Build history of the part. All positions in model axes, mm. Give positions to 0.01 mm unless a question says otherwise; leave off trailing zeros. Write each loop counter-clockwise with the first axis right and the second up, starting at its lowest first coordinate (ties: lowest second). Pieces come first, ordered by that corner, then holes. Notation, with made-up numbers: M 67.5,48 L 113.5,48 A27 ccw 113.5,80 Z; hole C 50.25,65 d8. An arc over 180 degrees is marked long. One line per item, written item: value. Start each with the question number.
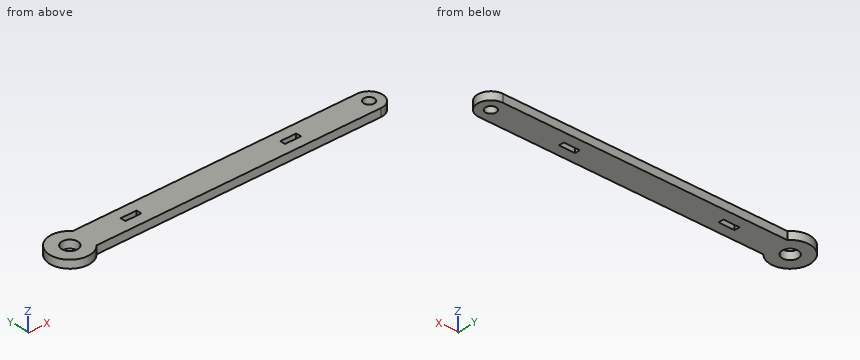
from build123d import *

# Parameters (mm, degrees)
SKETCH_1_R      = 2
SKETCH_1_R_2    = 3
SKETCH_1_W      = 6
SKETCH_1_H      = 2
EXTRUDE_1_DEPTH = 1.5


with BuildPart() as part:
    # 草图1 → 凸台-拉伸1 (new, symmetric)
    with BuildSketch(Plane.XY):
        with BuildLine():
            Line((5.590169944, 5), (112.5, 5))
            ThreePointArc((112.5, 5), (117.5, 0), (112.5, -5))
            Line((112.5, -5), (5.590169944, -5))
            ThreePointArc((5.590169944, -5), (-7.5, 0), (5.590169944, 5))
        make_face()
        with Locations((112.5, 0)):
            Circle(SKETCH_1_R, mode=Mode.SUBTRACT)
        Circle(SKETCH_1_R_2, mode=Mode.SUBTRACT)
        with Locations((23, 0)):
            Rectangle(SKETCH_1_W, SKETCH_1_H, mode=Mode.SUBTRACT)
        with Locations((83, 0)):
            Rectangle(SKETCH_1_W, SKETCH_1_H, mode=Mode.SUBTRACT)
    extrude(amount=EXTRUDE_1_DEPTH, both=True)


solid = part.part
1) Drop flat-ended pins along their axis: P1, Ø0.9, axis at x = 23, z = 0, coming from the -Y side; P2, Ø0.6, axis at y = -0.5, z = -0.5, coming from the +X side; P3, Ø0.9, axis at x = 84, z = 0, coming from the +Y side. Give the stop position or say it passes through.
2) Probe line 1 along Y through (x, z) = (112.5, 0.1); line 2 along Y through (x, z) = (0, 0.2); line 3 along X through (y, z) = (-1.25, 1.05). List the from-to ranges inside material, lowest first. Write a range as from..to.
3) Band-saw the part on B-B (z = -0.35). List the corners of the cut face in (x, y).
4) Band-saw the part on C-C (x = 14.5). List the corners of the cut face in (y, z).
5) Band-saw the part on A-A (x = 0). List the corners of the cut face in (y, z), then the cut area to 3 significant figures.
Model answer:
1. P1: stops at y = -5
1. P2: stops at x = 117.5
1. P3: stops at y = 5
2. line 1: y = -5..-2, 2..5
2. line 2: y = -7.5..-3, 3..7.5
2. line 3: x = -7.4..-2.73, 2.73..110.94, 114.06..117.34
3. outline: M 5.59,-5 L 112.5,-5 A5 ccw 112.5,5 L 5.59,5 A7.5 ccw long Z; hole C 0,0 d6; hole M 20,-1 L 26,-1 L 26,1 L 20,1 Z; hole M 80,-1 L 86,-1 L 86,1 L 80,1 Z; hole C 112.5,0 d4
4. outline: M -5,-1.5 L 5,-1.5 L 5,1.5 L -5,1.5 Z
5. outline: M -7.5,-1.5 L -3,-1.5 L -3,1.5 L -7.5,1.5 Z; M 3,-1.5 L 7.5,-1.5 L 7.5,1.5 L 3,1.5 Z
5. area: 27.0 mm²
